from build123d import *

# Parameters (mm, degrees)
F0_W     = 80
F0_H     = 20
F1_DEPTH = 390.5
F2_W     = 781
F2_H     = 163
F3_DEPTH = 5
F4_W     = 714
F4_H     = 124
F5_DEPTH = 5


with BuildPart() as f1:
    # F0 (on Right) → F1 (new body, symmetric)
    with BuildSketch(Plane.YZ):
        Polygon((-92.5, 50), (-92.5, 0), (-71.5, 0), (-71.5, 4), (-75.5, 4), (-75.5, 8), (-63.5, 8), (-63.5, 4), (-67.5, 4), (-67.5, 0), (-40, 0), (40, 0), (67.5, 0), (67.5, 4), (63.5, 4), (63.5, 8), (75.5, 8), (75.5, 4), (71.5, 4), (71.5, 0), (92.5, 0), (92.5, 50), align=None)
        with Locations((0, -10)):
            Rectangle(F0_W, F0_H)
    extrude(amount=F1_DEPTH, both=True)

    # F2 (on face) → F3 (cut)
    with BuildSketch(Plane.XY.offset(50)):
        Rectangle(F2_W, F2_H)
    extrude(amount=-F3_DEPTH, mode=Mode.SUBTRACT)

    # F4 (on face) → F5 (join)
    with BuildSketch(Plane.XY.offset(45)):
        with Locations((-13.5, 19.3)):
            Rectangle(F4_W, F4_H)
    extrude(amount=F5_DEPTH)


solid = f1.part
CAD build for the part. Positions are in the model's coordinates, mm. A direction names the side the tool comes from. Coordinates: 2 decimals unless noted, no trailing zeros.
Item 1: Pin check, flat tips, straight feed: pin 1 Ø6.5 at (x, y) = (20, -77) entering from -Z; pin 2 Ø3 at (x, z) = (-210, -5) entering from +Y; pin 3 Ø1.5 at (y, z) = (17.5, 48) entering from -X. Stop position of each tip, or through.
Check sheet entries:
pin 1: stops at z = 0
pin 2: stops at y = 40
pin 3: stops at x = -370.5
Item 2: Two-plate mould, pull along Y, no slides. Class faces 4 (the face through (27, -48, 45)), 5 (the face through (-390.5, -1, 15)), 6 (the face through (5, 40, -10)): +Y half, -Y half, draft (parallel to the pull), parting line (faces both ways), or undercut.
Check sheet entries:
face 4: undercut
face 5: draft
face 6: +Y half
Item 3: Drill centre lines: L1, parallel to Y at x = 187, z = 5.5; L2, parallel to Z at x = 243.5, y = -52.5; L3, parallel to Z at x = -182, y = -84. Where is each one in solid material? Low to high.
Check sheet entries:
L1: y = -92.5 to -75.5, -63.5 to 63.5, 75.5 to 92.5
L2: z = 0 to 45
L3: z = 0 to 50
Item 4: 3-axis set-ups, long thin cutter, end or side, ignore diameter. For faces 1 (the face through (5, 82, 0)), 2 (the face through (5, -82, 0)), 3 (the face through (-18, 20, 50)): which of +Z, -Z, +X, -X, +Y, -Y reach the whole face in a straight line?
Check sheet entries:
face 1: -Z, +X, -X, +Y
face 2: -Z, +X, -X, -Y
face 3: +Z, +X, -X, +Y, -Y
